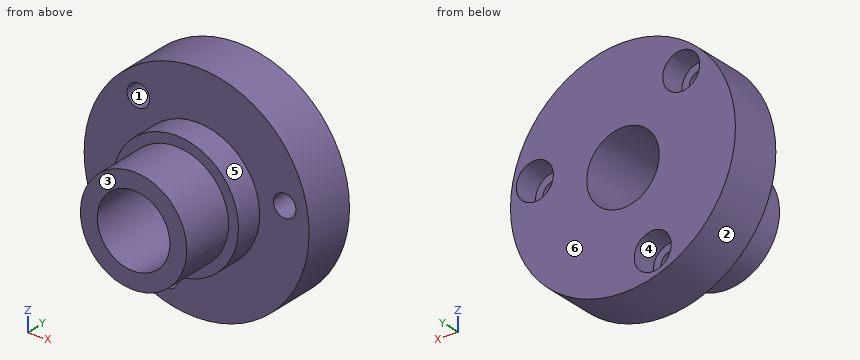
from build123d import *

# Parameters (mm, degrees)
F2_R     = 3.1
F2_R_2   = 10
F3_DEPTH = 47.8
F2_R_3   = 5.1
F4_DEPTH = 6.9


with BuildPart() as f1:
    # F0 (on Right) → F1 (revolve)
    with BuildSketch(Plane.YZ):
        Polygon((-22.1, 14.65), (-37.1, 14.65), (-37.1, 0), (0, 0), (0, 31), (-14.5, 31), (-14.5, 17.375), (-22.1, 17.375), align=None)
    revolve(axis=Axis((0, -18.55, 0), (0, -1, 0)))

    # F2 (on face) → F3 (cut)
    with BuildSketch(Plane(origin=(0, 0, 0), x_dir=(-1, 0, 0), z_dir=(0, 1, 0))):
        with Locations((-24.279309, 4.539293)):
            Circle(F2_R)
        Circle(F2_R_2)
        with Locations((16.070797, 18.756852)):
            Circle(F2_R)
        with Locations((8.208512, -23.296144)):
            Circle(F2_R)
    extrude(amount=-F3_DEPTH, mode=Mode.SUBTRACT)

    # F2 (on face) → F4 (cut)
    with BuildSketch(Plane(origin=(0, 0, 0), x_dir=(-1, 0, 0), z_dir=(0, 1, 0))):
        with Locations((-24.279309, 4.539293)):
            Circle(F2_R_3)
        with Locations((-24.279309, 4.539293)):
            Circle(F2_R, mode=Mode.SUBTRACT)
        with Locations((16.070797, 18.756852)):
            Circle(F2_R_3)
        with Locations((16.070797, 18.756852)):
            Circle(F2_R, mode=Mode.SUBTRACT)
        with Locations((8.208512, -23.296144)):
            Circle(F2_R_3)
        with Locations((8.208512, -23.296144)):
            Circle(F2_R, mode=Mode.SUBTRACT)
    extrude(amount=-F4_DEPTH, mode=Mode.SUBTRACT)


solid = f1.part
Build history of the part. All positions in model axes, mm. Face numbers are marked on the shaded views. A direction names the side the tool comes from. Coordinates: 2 decimals unless noted, no trailing zeros. Order: outer loops, then holes, each group sorted by start corner. A loop starts at its lowest first (then second) coordinate and runs counter-clockwise, first axis right, second up. Notation, with made-up numbers: (89, 63.5) -> (146, 63.5) arc R21 ccw to (146, 68.5) -> close; hole circle Ø3 at (20, 74.25). An arc over 180 degrees is marked (long way). One line per item, written item: value.
(1) Mould opens along Z. For the marked faces 1, 2 and 3 say: pulls with the +Z half, pulls with the -Z half, needs draft (parallel to the pull), parting line crosses it, or undercut.
Checked values:
face 1: undercut
face 2: parting line crosses it
face 3: needs draft
(2) Slice it at A-A, the plane x = 0. List the corners of the cut face in (y, z) (3 decimals), plus the area to 3 significant figures.
Checked values:
outline: (-37.1, -14.65) -> (-22.1, -14.65) -> (-22.1, -17.375) -> (-14.5, -17.375) -> (-14.5, -31) -> (0, -31) -> (0, -10) -> (-37.1, -10) -> close; (-37.1, 10) -> (0, 10) -> (0, 31) -> (-14.5, 31) -> (-14.5, 17.375) -> (-22.1, 17.375) -> (-22.1, 14.65) -> (-37.1, 14.65) -> close
area: 861 mm2
(3) Probe line 1 (Z direction, x = -6, y = -14); line 2 (Z direction, x = 0, y = -27); line 3 (Y direction, x = 0, z = 26). List the from-to ranges inside material, lowest first. Write a range as [from, to].
Checked values:
line 1: [-30.41, -25.47], [-21.12, -8], [8, 30.41]
line 2: [-14.65, -10], [10, 14.65]
line 3: [-14.5, 0]
(4) Drop flat-ended pins along their axis: pin 1 Ø5 at (x, z) = (24.28, 4.54) entering from -Y; pin 2 Ø3 at (x, y) = (-14.5, -4.5) entering from -Z; pin 3 Ø4 at (x, y) = (-8.5, -31) entering from +Z; pin 4 Ø3 at (x, z) = (-6.5, -21) entering from +Y. Give the stop position or say it passes through.
Checked values:
pin 1: through
pin 2: z = -28.14
pin 3: z = 13.13
pin 4: y = -6.9
(5) Slice it at D-D, the plane x = -9. List the corners of the cut face in (y, z).
Checked values:
outline: (-37.1, -11.56) -> (-22.1, -11.56) -> (-22.1, -14.86) -> (-14.5, -14.86) -> (-14.5, -20.3) -> (-6.9, -20.3) -> (-6.9, -18.26) -> (0, -18.26) -> (0, -4.36) -> (-37.1, -4.36) -> close; (-37.1, 4.36) -> (0, 4.36) -> (0, 29.66) -> (-14.5, 29.66) -> (-14.5, 14.86) -> (-22.1, 14.86) -> (-22.1, 11.56) -> (-37.1, 11.56) -> close; (-14.5, -29.66) -> (0, -29.66) -> (0, -28.33) -> (-6.9, -28.33) -> (-6.9, -26.29) -> (-14.5, -26.29) -> close
(6) Slice it at C-C, the plane y = -24. List the corners of the cut face in (x, z).
Checked values:
outline: circle Ø29.3 at (0, 0); hole circle Ø20 at (0, 0)
(7) Slice it at B-B, the plane z = 6.5. List the corners of the cut face in (x, y).
Checked values:
outline: (-30.31, -14.5) -> (-16.11, -14.5) -> (-16.11, -22.1) -> (-13.13, -22.1) -> (-13.13, -37.1) -> (-7.6, -37.1) -> (-7.6, 0) -> (-30.31, 0) -> close; (7.6, -37.1) -> (13.13, -37.1) -> (13.13, -22.1) -> (16.11, -22.1) -> (16.11, -14.5) -> (21.88, -14.5) -> (21.88, -6.9) -> (19.57, -6.9) -> (19.57, 0) -> (7.6, 0) -> close; (26.68, -14.5) -> (30.31, -14.5) -> (30.31, 0) -> (28.99, 0) -> (28.99, -6.9) -> (26.68, -6.9) -> close
(8) Tool access for the marked faces 4, 5 and 6: list every direction of +Z, -Z, +X, -X, +Y, -Y with a clear straight run to the whole face (end or side of a thin tool).
Checked values:
face 4: +Y
face 5: -Y
face 6: +Z, -Z, +X, -X, +Y
